Could you check a few things on this model? Use its own coordinates, in mm. Face numbers are marked on the shaded views. A direction names the side the tool comes from. Coordinates: 2 decimals unless noted, no trailing zeros. Loops run counter-clockwise (first coordinate to the right, second up) from the corner with the lowest first, then second, coordinate; pieces in that order, holes last. Notation, with made-up numbers: (-4.5, -37.5) -> (32.5, -37.5) arc R23 cw to (32.5, -15.5) -> close; hole circle Ø7 at (47, -23). An arc over 180 degrees is marked (long way). One line per question, with ' | ' between items.
from build123d import *

# Parameters (mm, degrees)
SKETCH1_W           = 60
SKETCH1_H           = 30
BOSS_EXTRUDE1_DEPTH = 2
SKETCH2_R           = 4
CUT_EXTRUDE1_DEPTH  = 13
SKETCH3_W           = 25
SKETCH3_H           = 15
CUT_EXTRUDE2_DEPTH  = 34.600595233
BOSS_EXTRUDE2_START = 1
SKETCH5_R           = 5
SKETCH5_R_2         = 4
BOSS_EXTRUDE2_DEPTH = 1
SKETCH7_R           = 5
SKETCH7_R_2         = 4
BOSS_EXTRUDE3_DEPTH = 1
SKETCH9_W           = 10
SKETCH9_H           = 4
BOSS_EXTRUDE4_DEPTH = 10
SKETCH10_R          = 2.25
CUT_EXTRUDE3_DEPTH  = 41.853396432
SKETCH11_R          = 2.25
CUT_EXTRUDE4_DEPTH  = 43.755116653
SKETCH13_W          = 14
SKETCH13_H          = 4
CUT_EXTRUDE6_DEPTH  = 36


with BuildPart() as part:
    # Sketch1 → Boss-Extrude1 (new body)
    with BuildSketch(Plane.XY):
        Rectangle(SKETCH1_W, SKETCH1_H)
    extrude(amount=BOSS_EXTRUDE1_DEPTH)

    # Sketch2 → Cut-Extrude1 (cut)
    with BuildSketch(Plane.XY.offset(2)):
        with Locations((-21, 3)):
            Circle(SKETCH2_R)
        with Locations((21, 3)):
            Circle(SKETCH2_R)
    extrude(amount=-CUT_EXTRUDE1_DEPTH, mode=Mode.SUBTRACT)

    # Sketch3 → Cut-Extrude2 (cut, through all)
    with BuildSketch(Plane.XY.offset(2)):
        with Locations((0, 2.5)):
            Rectangle(SKETCH3_W, SKETCH3_H)
    extrude(amount=-CUT_EXTRUDE2_DEPTH, mode=Mode.SUBTRACT)

    # Sketch5 → Boss-Extrude2 (add)
    # profile 1 of 2: a face of its own
    with BuildSketch(Plane.XY.offset(2).offset(BOSS_EXTRUDE2_START)):
        with Locations(Location((-21, 3, 0), (0, 0, 180))):
            Circle(SKETCH5_R)
        with Locations((-21, 3)):
            Circle(SKETCH5_R_2, mode=Mode.SUBTRACT)
    # profile 2 of 2: a face of its own
    with BuildSketch(Plane.XY.offset(2).offset(BOSS_EXTRUDE2_START)):
        with Locations(Location((21, 3, 0), (0, 0, 180))):
            Circle(SKETCH5_R)
        with Locations((21, 3)):
            Circle(SKETCH5_R_2, mode=Mode.SUBTRACT)
    extrude(amount=-BOSS_EXTRUDE2_DEPTH)

    # Sketch7 → Boss-Extrude3 (add)
    # profile 1 of 2: a face of its own
    with BuildSketch(Plane(origin=(0, 0, 0), x_dir=(-1, 0, 0), z_dir=(0, 0, -1))):
        with Locations((-21, 3)):
            Circle(SKETCH7_R)
        with Locations(Location((-21, 3, 0), (0, 0, 180))):
            Circle(SKETCH7_R_2, mode=Mode.SUBTRACT)
    # profile 2 of 2: a face of its own
    with BuildSketch(Plane(origin=(0, 0, 0), x_dir=(-1, 0, 0), z_dir=(0, 0, -1))):
        with Locations((21, 3)):
            Circle(SKETCH7_R)
        with Locations(Location((21, 3, 0), (0, 0, 180))):
            Circle(SKETCH7_R_2, mode=Mode.SUBTRACT)
    extrude(amount=BOSS_EXTRUDE3_DEPTH)

    # Sketch9 → Boss-Extrude4 (add)
    with BuildSketch(Plane.XY.offset(2)):
        with Locations((0, -11)):
            Rectangle(SKETCH9_W, SKETCH9_H)
        with Locations((0, 12)):
            Rectangle(SKETCH9_W, SKETCH9_H)
    extrude(amount=BOSS_EXTRUDE4_DEPTH)

    # Sketch10 → Cut-Extrude3 (cut, through all)
    with BuildSketch(Plane.XZ.offset(-10)):
        with Locations((0, 7)):
            Circle(SKETCH10_R)
    extrude(amount=-CUT_EXTRUDE3_DEPTH, mode=Mode.SUBTRACT)

    # Sketch11 → Cut-Extrude4 (cut, through all)
    with BuildSketch(Plane.XZ.offset(13)):
        with Locations((0, 7)):
            Circle(SKETCH11_R)
    extrude(amount=-CUT_EXTRUDE4_DEPTH, mode=Mode.SUBTRACT)

    # Sketch13 → Cut-Extrude6 (cut, through all)
    with BuildSketch(Plane.XY.offset(2)):
        with Locations((0, -7)):
            Rectangle(SKETCH13_W, SKETCH13_H)
    extrude(amount=-CUT_EXTRUDE6_DEPTH, mode=Mode.SUBTRACT)


solid = part.part
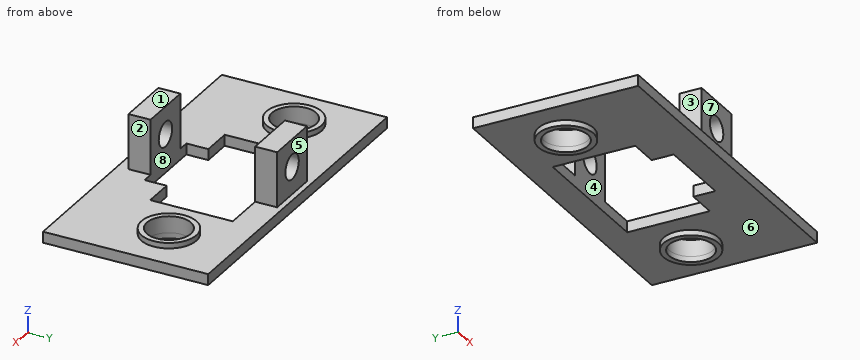
1) If we section it at C-C on z = 7: Please give me the cut outline in (x, y), and give its area (3 significant figures).
Data:
outline: (-5, -13) -> (-2.25, -13) -> (-2.25, -9) -> (-5, -9) -> close; (-5, 10) -> (-2.25, 10) -> (-2.25, 14) -> (-5, 14) -> close; (2.25, -13) -> (5, -13) -> (5, -9) -> (2.25, -9) -> close; (2.25, 10) -> (5, 10) -> (5, 14) -> (2.25, 14) -> close | area: 44.0 mm²
2) I need wall thicknesses on line 1 along Y through (x, z) = (-21, 1.05); line 2 along Z through (x, y) = (0, 12.3); line 3 along Y through (x, z) = (21, -0.25). Which ranges of each line are inside material? Lowest first, please. Write a range as from..to.
Data:
line 1: -15..-1, 7..15 | line 2: 0..4.75, 9.25..12 | line 3: -2..-1, 7..8
3) If we section it at A-A on y = -3.5: Please give me the cut outline in (x, z), and give its area (3 significant figures).
Data:
outline: (-30, 0) -> (-12.5, 0) -> (-12.5, 2) -> (-30, 2) -> close; (12.5, 0) -> (30, 0) -> (30, 2) -> (12.5, 2) -> close | area: 70.0 mm²
4) We'd pull the mould along Y, two halves only. Please class the marked faces 6, 7 and 8: pulls with the +Y half, pulls with the -Y half, needs draft (parallel to the pull), parting line crosses it, or undercut.
Data:
face 6: needs draft | face 7: pulls with the -Y half | face 8: undercut
5) I'm going to push flat-ended pins straight in: pin 1 Ø3 at (x, z) = (0, 6.5) entering from +Y; pin 2 Ø2 at (y, z) = (-11, 7) entering from +X; pin 3 Ø5 at (x, z) = (0, 8) entering from -Y; pin 4 Ø15 at (x, y) = (-11.5, 0.5) entering from +Z. Where does each tip first touch, or does it pass through?
Data:
pin 1: through | pin 2: x = 5 | pin 3: y = -13 | pin 4: z = 3
6) If we section it at D-D on x = 21: Please give me the cut outline in (y, z), and give its area (3 significant figures).
Data:
outline: (-15, 0) -> (-2, 0) -> (-2, -1) -> (-1, -1) -> (-1, 3) -> (-2, 3) -> (-2, 2) -> (-15, 2) -> close; (7, -1) -> (8, -1) -> (8, 0) -> (15, 0) -> (15, 2) -> (8, 2) -> (8, 3) -> (7, 3) -> close | area: 48.0 mm²
7) On a 3-axis mill with a long thin cutter (end or side, diameter ignored), from which of +Z, -Z, +X, -X, +Y, -Y can I reach the whole of each face in a straight line? I mean the marked faces 1, 2, 3, 4 and 5. Say none if no direction works.
Data:
face 1: +Z, +X, -X, +Y, -Y | face 2: +Z, +X, +Y, -Y | face 3: +Z, -X, +Y, -Y | face 4: +Z, -Z | face 5: +Z, +X, -X, +Y
8) If we section it at B-B on x = 0: Please give me the cut outline in (y, z), and give its area (3 significant figures).
Data:
outline: (-15, 0) -> (-9, 0) -> (-9, 4.75) -> (-13, 4.75) -> (-13, 2) -> (-15, 2) -> close; (-13, 9.25) -> (-9, 9.25) -> (-9, 12) -> (-13, 12) -> close; (10, 0) -> (15, 0) -> (15, 2) -> (14, 2) -> (14, 4.75) -> (10, 4.75) -> close; (10, 9.25) -> (14, 9.25) -> (14, 12) -> (10, 12) -> close | area: 66.0 mm²
